Read the model definition and answer for the solid it produces. Units are mm, in the model's axes. Face numbers are marked on the shaded views. Coordinates: 2 decimals unless noted, no trailing zeros. Write each loop counter-clockwise with the first axis right and the second up, starting at its lowest first coordinate (ties: lowest second). Pieces come first, ordered by that corner, then holes.
1) This flat-tipped pin is pushed along its axis until it touches: pin 1 Ø4 at (x, y) = (22.86, 0) entering from -Z. Where does it stop, or does it pass through?
2) Determine the mould class of the marked faces 1, 2 and 3 for opening direction Y: +Y half, -Y half, draft (parallel to the pull), parting line (faces both ways), or undercut.
3) The part is cut by section C-C (x = -22.86). Determine the outline of the cut face in (y, z) (3 decimals).
4) The part is cut by section D-D (z = -8). Determine the outline of the cut face in (x, y) (3 decimals), then the cut area to 3 significant figures.
5) Find the intervals of material crossed by line 1 (X direction, y = -2.5, z = -8.25) (3 decimals); line 2 (X direction, y = -1, z = -3.5) (3 decimals); line 3 (Y direction, x = -22.86, z = -2.75) (3 decimals), in increasing order.
6) The part is cut by section A-A (z = -5.75). Determine the outline of the cut face in (x, y) (3 decimals), then the cut area to 3 significant figures.
7) The part is cut by section B-B (y = 0). Determine the outline of the cut face in (x, z) (3 decimals), then the cut area to 3 significant figures.
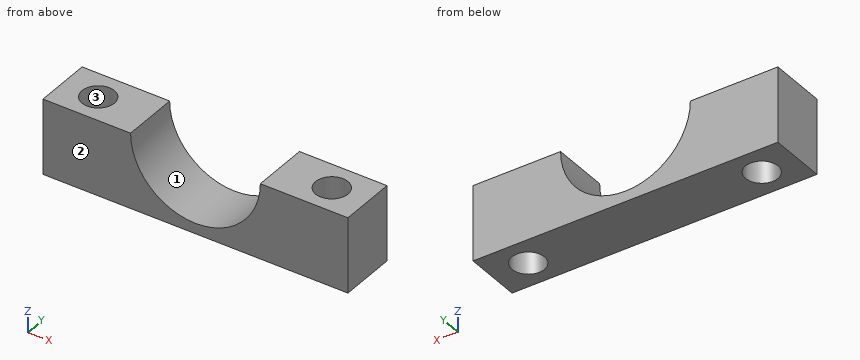
from build123d import *

# Parameters (mm, degrees)
BOSS_EXTRUDE1_DEPTH = 5.5626
SKETCH2_R           = 3.175
CUT_EXTRUDE1_DEPTH  = 34.744605017


with BuildPart() as part:
    # Sketch1 → Boss-Extrude1 (new, symmetric)
    with BuildSketch(Plane(origin=(0, 0, 0), x_dir=(1, 0, 0), z_dir=(0, 1, 0))):
        with BuildLine():
            Line((-12.7, 0), (-29.845, 0))
            Line((-29.845, 0), (-29.845, 14.732))
            Line((-29.845, 14.732), (29.845, 14.732))
            Line((29.845, 14.732), (29.845, 0))
            Line((29.845, 0), (12.7, 0))
            ThreePointArc((12.7, 0), (0, 12.7), (-12.7, 0))
        make_face()
    extrude(amount=BOSS_EXTRUDE1_DEPTH, both=True)

    # Sketch2 → Cut-Extrude1 (cut, through all)
    with BuildSketch(Plane.XY):
        with Locations((-22.86, 0)):
            Circle(SKETCH2_R)
        with Locations((22.86, 0)):
            Circle(SKETCH2_R)
    extrude(amount=-CUT_EXTRUDE1_DEPTH, mode=Mode.SUBTRACT)


solid = part.part
Reported:
1. pin 1: passes through
2. face 1: draft
2. face 2: -Y half
2. face 3: undercut
3. outline: (-5.563, -14.732) - (-3.175, -14.732) - (-3.175, 0) - (-5.563, 0) - close; (3.175, -14.732) - (5.563, -14.732) - (5.563, 0) - (3.175, 0) - close
4. outline: (-29.845, -5.563) - (-9.864, -5.563) - (-9.864, 5.563) - (-29.845, 5.563) - close; (9.864, -5.563) - (29.845, -5.563) - (29.845, 5.563) - (9.864, 5.563) - close; hole circle Ø6.35 at (-22.86, 0); hole circle Ø6.35 at (22.86, 0)
4. area: 381 mm2
5. line 1: x = -29.845 to -24.817, -20.903 to -9.655, 9.655 to 20.903, 24.817 to 29.845
5. line 2: x = -29.845 to -25.873, -19.847 to -12.208, 12.208 to 19.847, 25.873 to 29.845
5. line 3: y = -5.563 to -3.175, 3.175 to 5.563
6. outline: (-29.845, -5.563) - (-11.324, -5.563) - (-11.324, 5.563) - (-29.845, 5.563) - close; (11.324, -5.563) - (29.845, -5.563) - (29.845, 5.563) - (11.324, 5.563) - close; hole circle Ø6.35 at (-22.86, 0); hole circle Ø6.35 at (22.86, 0)
6. area: 349 mm2
7. outline: (-29.845, -14.732) - (-26.035, -14.732) - (-26.035, 0) - (-29.845, 0) - close; (-19.685, -14.732) - (19.685, -14.732) - (19.685, 0) - (12.7, 0) arc R12.7 cw to (-12.7, 0) - (-19.685, 0) - close; (26.035, -14.732) - (29.845, -14.732) - (29.845, 0) - (26.035, 0) - close
7. area: 439 mm2
